Autodesk Inventor part; units mm, degrees
ref_plane "YZ Plane" through (0, 0, 0) normal (1, 0, 0) x (0, 1, 0)
ref_plane "XZ Plane" through (0, 0, 0) normal (0, 1, 0) x (-1, 0, 0)
ref_plane "XY Plane" through (0, 0, 0) normal (0, 0, 1) x (1, 0, 0)
sketch "Sketch1" plane through (0, 0, 0) normal (0, 1, 0) x (-1, 0, 0)
  circle A0 centre (0, 0) radius 80 construction
  line L0 (56.002, 57.1295) -> (-56.002, 57.1295) construction
  line L1 (-56.002, 57.1295) -> (-56.002, -57.1295) construction
  line L2 (-56.002, -57.1295) -> (56.002, -57.1295) construction
  line L3 (56.002, -57.1295) -> (56.002, 57.1295) construction
  line L4 (56.002, 57.1295) -> (-56.002, -57.1295) construction
  line L5 (-56.002, 57.1295) -> (56.002, -57.1295) construction
  line L6 (54.002, 55.1295) -> (-54.002, 55.1295)
  line L7 (-54.002, 55.1295) -> (-54.002, -55.1295)
  line L8 (-54.002, -55.1295) -> (54.002, -55.1295)
  line L9 (54.002, -55.1295) -> (54.002, 55.1295)
  dimension "d0" = 160
  dimension "d1" = 2
extrude "Extrusion1" add sketch "Sketch1" along normal blind 2
sketch "Sketch2" plane through (0, 0, 0) normal (0, -1, 0) x (1, 0, 0)
  line L0 (-39.0523, 32.251) -> (-42.2277, 32.251) construction
  line L1 (-42.2277, 32.251) -> (-43.8154, 35.001) construction
  line L2 (-43.8154, 35.001) -> (-42.2277, 37.751) construction
  line L3 (-42.2277, 37.751) -> (-39.0523, 37.751) construction
  line L4 (-39.0523, 37.751) -> (-37.4646, 35.001) construction
  line L5 (-37.4646, 35.001) -> (-39.0523, 32.251) construction
  line L6 (42.2277, 32.251) -> (39.0523, 32.251) construction
  line L7 (39.0523, 32.251) -> (37.4646, 35.001) construction
  line L8 (37.4646, 35.001) -> (39.0523, 37.751) construction
  line L9 (39.0523, 37.751) -> (42.2277, 37.751) construction
  line L10 (42.2277, 37.751) -> (43.8154, 35.001) construction
  line L11 (43.8154, 35.001) -> (42.2277, 32.251) construction
  line L12 (48.9587, -27.749) -> (45.7833, -27.749) construction
  line L13 (45.7833, -27.749) -> (44.1956, -24.999) construction
  line L14 (44.1956, -24.999) -> (45.7833, -22.249) construction
  line L15 (45.7833, -22.249) -> (48.9587, -22.249) construction
  line L16 (48.9587, -22.249) -> (50.5464, -24.999) construction
  line L17 (50.5464, -24.999) -> (48.9587, -27.749) construction
  line L18 (-45.7833, -22.249) -> (-44.1956, -24.999) construction
  line L19 (-44.1956, -24.999) -> (-45.7833, -27.749) construction
  line L20 (-45.7833, -27.749) -> (-48.9587, -27.749) construction
  line L21 (-48.9587, -27.749) -> (-50.5464, -24.999) construction
  line L22 (-50.5464, -24.999) -> (-48.9587, -22.249) construction
  line L23 (-48.9587, -22.249) -> (-45.7833, -22.249) construction
  line L24 (-47.371, -24.999) -> (47.371, -24.999) construction
  line L25 (-40.64, 35.001) -> (40.64, 35.001) construction
  line L26 (-75.6027, 0) -> (75.6027, 0) construction
  line L27 (0, -77.1813) -> (0, 77.1813) construction
  line L28 (-37.3491, 35.001) -> (-38.9946, 37.851)
  line L29 (-38.9946, 37.851) -> (-42.2854, 37.851)
  line L30 (-42.2854, 37.851) -> (-43.9309, 35.001)
  line L31 (-43.9309, 35.001) -> (-42.2854, 32.151)
  line L32 (-42.2854, 32.151) -> (-38.9946, 32.151)
  line L33 (-38.9946, 32.151) -> (-37.3491, 35.001)
  line L34 (49.0164, -27.849) -> (45.7256, -27.849)
  line L35 (45.7256, -27.849) -> (44.0801, -24.999)
  line L36 (44.0801, -24.999) -> (45.7256, -22.149)
  line L37 (45.7256, -22.149) -> (49.0164, -22.149)
  line L38 (49.0164, -22.149) -> (50.6619, -24.999)
  line L39 (50.6619, -24.999) -> (49.0164, -27.849)
  line L40 (43.9309, 35.001) -> (42.2854, 37.851)
  line L41 (42.2854, 37.851) -> (38.9946, 37.851)
  line L42 (38.9946, 37.851) -> (37.3491, 35.001)
  line L43 (37.3491, 35.001) -> (38.9946, 32.151)
  line L44 (38.9946, 32.151) -> (42.2854, 32.151)
  line L45 (42.2854, 32.151) -> (43.9309, 35.001)
  line L46 (-45.7256, -27.849) -> (-44.0801, -24.999)
  line L47 (-44.0801, -24.999) -> (-45.7256, -22.149)
  line L48 (-45.7256, -22.149) -> (-49.0164, -22.149)
  line L49 (-49.0164, -22.149) -> (-50.6619, -24.999)
  line L50 (-50.6619, -24.999) -> (-49.0164, -27.849)
  line L51 (-49.0164, -27.849) -> (-45.7256, -27.849)
  line L52 (-35.0397, 35.001) -> (-37.8399, 39.851)
  line L53 (-37.8399, 39.851) -> (-43.4401, 39.851)
  line L54 (-43.4401, 39.851) -> (-46.2403, 35.001)
  line L55 (-46.2403, 35.001) -> (-43.4401, 30.151)
  line L56 (-43.4401, 30.151) -> (-37.8399, 30.151)
  line L57 (-37.8399, 30.151) -> (-35.0397, 35.001)
  line L58 (46.2403, 35.001) -> (43.4401, 39.851)
  line L59 (43.4401, 39.851) -> (37.8399, 39.851)
  line L60 (37.8399, 39.851) -> (35.0397, 35.001)
  line L61 (35.0397, 35.001) -> (37.8399, 30.151)
  line L62 (37.8399, 30.151) -> (43.4401, 30.151)
  line L63 (43.4401, 30.151) -> (46.2403, 35.001)
  line L64 (44.5709, -29.849) -> (50.1711, -29.849)
  line L65 (50.1711, -29.849) -> (52.9713, -24.999)
  line L66 (52.9713, -24.999) -> (50.1711, -20.149)
  line L67 (50.1711, -20.149) -> (44.5709, -20.149)
  line L68 (44.5709, -20.149) -> (41.7707, -24.999)
  line L69 (41.7707, -24.999) -> (44.5709, -29.849)
  line L70 (-44.5709, -29.849) -> (-41.7707, -24.999)
  line L71 (-41.7707, -24.999) -> (-44.5709, -20.149)
  line L72 (-44.5709, -20.149) -> (-50.1711, -20.149)
  line L73 (-50.1711, -20.149) -> (-52.9713, -24.999)
  line L74 (-52.9713, -24.999) -> (-50.1711, -29.849)
  line L75 (-50.1711, -29.849) -> (-44.5709, -29.849)
  point P0 (0, 0)
  point P1 (0, 35.001)
  point P2 (0, -24.999)
  dimension "d4" = 5.5
  dimension "d5" = 5.5
  dimension "d6" = 5.5
  dimension "d7" = 5.5
  dimension "d8" = 81.28
  dimension "d9" = 94.742
  dimension "d10" = 24.999
  dimension "d11" = 35.001
  dimension "d12" = 0.1
  dimension "d13" = 0.1
  dimension "d14" = 0.1
  dimension "d15" = 0.1
  dimension "d16" = 2
  dimension "d17" = 2
  dimension "d18" = 2
  dimension "d19" = 2
extrude "Extrusion2" add sketch "Sketch2" along normal blind 5
sketch "Sketch3" plane through (0, 2, 0) normal (0, 1, 0) x (1, 0, 0)
  line L0 (-42.2854, -37.851) -> (-43.9309, -35.001) construction
  line L1 (-43.9309, -35.001) -> (-42.2854, -32.151) construction
  line L2 (-42.2854, -32.151) -> (-38.9946, -32.151) construction
  line L3 (-38.9946, -32.151) -> (-37.3491, -35.001) construction
  line L4 (-37.3491, -35.001) -> (-38.9946, -37.851) construction
  line L5 (-38.9946, -37.851) -> (-42.2854, -37.851) construction
  line L6 (-50.6619, 24.999) -> (-49.0164, 27.849) construction
  line L7 (-49.0164, 27.849) -> (-45.7256, 27.849) construction
  line L8 (-45.7256, 27.849) -> (-44.0801, 24.999) construction
  line L9 (-44.0801, 24.999) -> (-45.7256, 22.149) construction
  line L10 (-45.7256, 22.149) -> (-49.0164, 22.149) construction
  line L11 (-49.0164, 22.149) -> (-50.6619, 24.999) construction
  line L12 (50.6619, 24.999) -> (49.0164, 22.149) construction
  line L13 (49.0164, 22.149) -> (45.7256, 22.149) construction
  line L14 (45.7256, 22.149) -> (44.0801, 24.999) construction
  line L15 (44.0801, 24.999) -> (45.7256, 27.849) construction
  line L16 (45.7256, 27.849) -> (49.0164, 27.849) construction
  line L17 (49.0164, 27.849) -> (50.6619, 24.999) construction
  line L18 (42.2854, -32.151) -> (43.9309, -35.001) construction
  line L19 (43.9309, -35.001) -> (42.2854, -37.851) construction
  line L20 (42.2854, -37.851) -> (38.9946, -37.851) construction
  line L21 (38.9946, -37.851) -> (37.3491, -35.001) construction
  line L22 (37.3491, -35.001) -> (38.9946, -32.151) construction
  line L23 (38.9946, -32.151) -> (42.2854, -32.151) construction
  line L24 (47.371, 27.849) -> (47.371, 22.149) construction
  line L25 (49.0164, 22.149) -> (50.6619, 24.999) construction
  line L26 (-49.0164, 22.149) -> (-50.6619, 24.999) construction
  line L27 (50.6619, 24.999) -> (-50.6619, 24.999) construction
  line L28 (-49.0164, 27.849) -> (-45.7256, 27.849) construction
  line L29 (-47.371, 27.849) -> (-47.371, 22.149) construction
  line L30 (-45.7256, 22.149) -> (-49.0164, 22.149) construction
  line L31 (-38.9946, -37.851) -> (-42.2854, -37.851) construction
  line L32 (-40.64, -37.851) -> (-40.64, -32.151) construction
  line L33 (-43.9309, -35.001) -> (43.9309, -35.001) construction
  line L34 (38.9946, -32.151) -> (42.2854, -32.151) construction
  line L35 (40.64, -32.151) -> (40.64, -37.851) construction
  point P0 (0, 0)
  point P1 (-47.371, 24.999)
  point P2 (47.371, 24.999)
  point P3 (40.64, -35.001)
  point P4 (-40.64, -35.001)
hole "Hole1" at (-47.371, 2, -24.999) at (47.371, 2, -24.999) at (40.64, 2, 35.001) at (-40.64, 2, 35.001) direction (0, -1, 0) diameter 3.4 end through all countersink diameter 6.3 countersink angle 90
sketch "Sketch4" plane through (0, 2, 0) normal (0, 1, 0) x (1, 0, 0)
  circle A0 centre (47.371, 24.999) radius 3.15 construction
  circle A1 centre (-47.371, 24.999) radius 3.15 construction
  line L0 (54.002, 55.1295) -> (-54.002, 55.1295) construction
  circle A2 centre (40.64, -35.001) radius 3.15 construction
  circle A3 centre (-40.64, -35.001) radius 3.15 construction
  line L1 (-54.002, -55.1295) -> (54.002, -55.1295) construction
  circle A4 centre (-47.371, 24.999) radius 1.7 construction
  circle A5 centre (40.64, -35.001) radius 1.7 construction
  line L2 (-47.371, 24.999) -> (40.64, -35.001) construction
  line L3 (47.371, 24.999) -> (-40.64, -35.001) construction
  line L4 (-40.4554, 23.9152) -> (37.1041, -28.9597)
  line L5 (-43.8351, 18.9577) -> (33.7244, -33.9172)
  line L6 (43.8351, 18.9577) -> (-33.7244, -33.9172)
  line L7 (40.4554, 23.9152) -> (-37.1041, -28.9597)
  line L8 (-2.5, 48.1295) -> (2.5, 48.1295)
  line L9 (2.5, 48.1295) -> (2.5, -1.9602)
  line L10 (2.5, -1.9602) -> (-2.5, -1.9602)
  line L11 (-2.5, -1.9602) -> (-2.5, 48.1295)
  circle A6 centre (-47.371, 24.999) radius 7
  circle A7 centre (47.371, 24.999) radius 1.7
  circle A8 centre (47.371, 24.999) radius 7
  circle A9 centre (40.64, -35.001) radius 7
  circle A10 centre (-40.64, -35.001) radius 7
  circle A11 centre (40.64, -35.001) radius 3.15 construction
  circle A12 centre (-47.371, 24.999) radius 3.15 construction
  circle A13 centre (47.371, 24.999) radius 3.15 construction
  circle A14 centre (-40.64, -35.001) radius 3.15 construction
  line L12 (54.002, 55.1295) -> (-54.002, 55.1295) construction
  line L13 (-54.002, 55.1295) -> (-54.002, -55.1295) construction
  line L14 (-54.002, -55.1295) -> (54.002, -55.1295) construction
  line L15 (54.002, -55.1295) -> (54.002, 55.1295) construction
  line L16 (-47.002, -48.1295) -> (-47.002, 48.1295)
  line L17 (-47.002, 48.1295) -> (47.002, 48.1295)
  line L18 (47.002, 48.1295) -> (47.002, -48.1295)
  line L19 (47.002, -48.1295) -> (-47.002, -48.1295)
  line L20 (40.64, -28.001) -> (47.002, -28.001)
  line L21 (-40.64, -28.001) -> (-47.002, -28.001)
  line L22 (-33.64, -35.001) -> (-33.64, -48.1295)
  line L23 (33.64, -35.001) -> (33.64, -48.1295)
  point P0 (0, -10.9262)
  point P1 (5.3259, -7.2954)
  point P2 (-5.3259, -7.2954)
  point P3 (-47.002, 18.0087)
  point P4 (47.002, 18.0087)
  point P5 (47.002, 31.9893)
  point P6 (-47.002, 31.9893)
  dimension "d43" = 3
  dimension "d44" = 3
  dimension "d45" = 3
  dimension "d46" = 3
  dimension "d47" = 5
  dimension "d50" = 14
  dimension "d51" = 14
  dimension "d52" = 14
  dimension "d53" = 14
  dimension "d54" = 7
extrude "Extrusion3" cut sketch "Sketch4" against normal through all contours A6 L16 L17 L11 L4 | L5 L7 A10 L21 L16 A6 | L9 L17 L18 A8 L7 | L6 A8 L18 L20 A9 L4 | L5 A9 L23 L19 L22 A10 L6
equation "\"d5\" = d4"
equation "\"d6\" = d4"
equation "\"d7\" = d4"
equation "\"d17\" = d16"
equation "\"d18\" = d16"
equation "\"d19\" = d16"
equation "\"d44\" = d43"
equation "\"d45\" = d43"
equation "\"d46\" = d43"
equation "\"d50\" = 2 * d35"
equation "\"d51\" = 2 * d35"
equation "\"d52\" = 2 * d35"
equation "\"d53\" = 2 * d35"
equation "\"d54\" = d35"
equation "\"d39\" = d35"
properties part number "top_base"
Geometry: final body of the model. Coordinates: model frame, mm. A direction names the side the tool comes from. Round coordinates to 2 decimals unless told otherwise and drop trailing zeros. Order: outer loops, then holes, each group sorted by start corner. A loop starts at its lowest first (then second) coordinate and runs counter-clockwise, first axis right, second up. Notation, with made-up numbers: M 86,11.25 L 145,11.25 A18 ccw 145,39.25 Z; hole C 72,75 d1. An arc over 180 degrees is marked long. One line per item, written item: value.
(1) Pin query (flat end, axial travel): P1, Ø2.5, axis at x = -41, y = -2.5, coming from the -Z side; P2, Ø2, axis at y = -3, z = -23, coming from the -X side; P3, Ø1.5, axis at x = 48, y = -3, coming from the -Z side; P4, Ø2.5, axis at x = -40.64, z = 35.001, coming from the +Y side. Return the tip coordinate at first contact, or that it passes through.
Result sheet:
P1: z = -25.83
P2: x = -52.39
P3: z = -29.85
P4: through
(2) Reachability of faces 1 (the flat face through (44.82, -2.46, 32.54)), 2 (the flat face through (-44.86, -2.46, 32.61)), 3 (the flat face through (36.46, -2.46, 37.46)), 4 (the cylindrical face through (41.986, 1.014, -29.471)), 5 (the flat face through (-47, -2, -27.849)) from +Z, -Z, +X, -X, +Y, -Y: full face, straight path, thin tool, end or side. Return the list, or none.
Result sheet:
face 1: +X, -Y
face 2: -X, -Y
face 3: +Z, -Y
face 4: +Y, -Y
face 5: -Y
(3) Cut plane B-B (x = 19). Return the cut outline in (y, z).
Result sheet:
outline: M 0,-55.13 L 2,-55.13 L 2,-48.13 L 0,-48.13 Z; M 0,-9.29 L 2,-9.29 L 2,-2.03 L 0,-2.03 Z; M 0,16.62 L 2,16.62 L 2,23.88 L 0,23.88 Z; M 0,48.13 L 2,48.13 L 2,55.13 L 0,55.13 Z
(4) Pull-direction query (Z, two-part tool) for faces 6 (the flat face through (1, 2, 1)), 7 (the flat face through (21.743, 1.014, -11.159)), 8 (the flat face through (44.86, -2.46, 37.39)); classes: pulls with the +Z half, pulls with the -Z half, needs draft (parallel to the pull), parting line crosses it, or undercut.
Result sheet:
face 6: needs draft
face 7: undercut
face 8: pulls with the +Z half
(5) Cut plane A-A (z = -4.5). Return the cut outline in (x, y).
Result sheet:
outline: M -54,0 L -47,0 L -47,2 L -54,2 Z; M -22.63,0 L -11.98,0 L -11.98,2 L -22.63,2 Z; M -2.5,0 L 2.5,0 L 2.5,2 L -2.5,2 Z; M 11.98,0 L 22.63,0 L 22.63,2 L 11.98,2 Z; M 47,0 L 54,0 L 54,2 L 47,2 Z
(6) Line query: probe 1 along X at (y, z) = (0.25, -47); probe 2 along Z at (x, y) = (-13.5, 1.75); probe 3 along Z at (x, y) = (-43.5, 1.5). Output: solid intervals per line, ascending. Write a range as [from, to].
Result sheet:
probe 1: [-54, -47], [-2.5, 2.5], [47, 54]
probe 2: [-55.13, -48.13], [-5.54, 1.72], [12.87, 20.13], [48.13, 55.13]
probe 3: [-55.13, -48.13], [-30.83, -18.73], [28, 55.13]
